```python
from build123d import *

# Parameters (mm, degrees)
SKETCH_W              = 115
SKETCH_H              = 25
PAD_DEPTH             = 3
PAD001_DEPTH          = 3
SKETCH002_W           = 115
SKETCH002_H           = 25
SKETCH002_W_2         = 96
SKETCH002_H_2         = 3
PAD002_DEPTH          = 3
SKETCH003_R           = 0.825
POCKET_DEPTH          = 245.060315
POLARPATTERN_COUNT    = 2
POLARPATTERN001_COUNT = 2
POLARPATTERN002_COUNT = 2
FILLET_R              = 2
SKETCH004_R           = 12.75
POCKET001_DEPTH       = 3
POCKET002_DEPTH       = 3


with BuildPart() as part:
    # Sketch → Pad (new body)
    with BuildSketch(Plane.XY):
        Rectangle(SKETCH_W, SKETCH_H)
    extrude(amount=PAD_DEPTH)

    # Sketch001 (on Face6 of Pad) → Pad001 (join)
    with BuildSketch(Plane.XY.offset(3)):
        Polygon((-57.5, 12.5), (57.5, 12.5), (57.5, 4), (50, 4), (50, 5), (-50, 5), (-50, 4), (-57.5, 4), align=None)
        Polygon((-57.5, -12.5), (57.5, -12.5), (57.5, -4), (50, -4), (50, -5), (-50, -5), (-50, -4), (-57.5, -4), align=None)
    extrude(amount=PAD001_DEPTH)

    # Sketch002 (on Face12 of Pad001) → Pad002 (join)
    with BuildSketch(Plane.XY.offset(6)):
        Rectangle(SKETCH002_W, SKETCH002_H)
        Rectangle(SKETCH002_W_2, SKETCH002_H_2, mode=Mode.SUBTRACT)
    extrude(amount=PAD002_DEPTH)

    # Sketch003 (on Face26 of Pad002) → Pocket (cut, through all)
    with BuildSketch(Plane.XY.offset(9)):
        with Locations((-52.5, 7.5)):
            Circle(SKETCH003_R)
    pocket = extrude(amount=-POCKET_DEPTH, mode=Mode.SUBTRACT)

    # PolarPattern: Pocket ×2 about axis
    polarpattern_axis = Axis((0, 0, 0), (0, 1, 0))
    for i in range(1, POLARPATTERN_COUNT):
        add(pocket.rotate(polarpattern_axis, i * 360 / POLARPATTERN_COUNT), mode=Mode.SUBTRACT)

    # PolarPattern001: Pocket ×2 about axis
    polarpattern001_axis = Axis((0, 0, 0), (1, 0, 0))
    for i in range(1, POLARPATTERN001_COUNT):
        add(pocket.rotate(polarpattern001_axis, i * 360 / POLARPATTERN001_COUNT), mode=Mode.SUBTRACT)

    # PolarPattern002: Pocket ×2 about axis
    polarpattern002_axis = Axis((0, 0, 9), (0, 0, 1))
    for i in range(1, POLARPATTERN002_COUNT):
        add(pocket.rotate(polarpattern002_axis, i * 360 / POLARPATTERN002_COUNT), mode=Mode.SUBTRACT)

    # Fillet
    fillet_edges = [part.edges().sort_by_distance(p)[0] for p in [
        (57.5, 12.5, 7.5),
        (57.5, 12.5, 4.5),
        (57.5, 12.5, 1.5),
        (57.5, -12.5, 7.5),
        (-57.5, 12.5, 7.5),
        (-57.5, -12.5, 7.5),
    ]]
    fillet(fillet_edges, radius=FILLET_R)

    # Sketch004 (on Face2 of Fillet) → Pocket001 (cut)
    with BuildSketch(Plane(origin=(0, 0, 0), x_dir=(1, 0, 0), z_dir=(0, 0, -1))):
        with Locations((0, -4.31247)):
            Circle(SKETCH004_R)
    extrude(amount=-POCKET001_DEPTH, mode=Mode.SUBTRACT)

    # Sketch005 (on Face2 of Pocket001) → Pocket002 (cut)
    with BuildSketch(Plane(origin=(0, 0, 0), x_dir=(1, 0, 0), z_dir=(0, 0, -1))):
        Polygon((0.086598, 10.584693), (-49.736099, 10.584693), (-49.736099, 6.30074), (-54.94091, 3.161258), (-54.94091, -2.621142), (-51.300568, -2.835279), (-51.086433, 1.161956), (-44.025761, 5.729707), (0.086598, 5.729707), align=None)
    extrude(amount=-POCKET002_DEPTH, mode=Mode.SUBTRACT)


solid = part.part
```
The model under review builds one solid part; all positions refer to its coordinate system, in mm. A direction names the side the tool comes from. Coordinates: 2 decimals unless noted, no trailing zeros. Write each loop counter-clockwise with the first axis right and the second up, starting at its lowest first coordinate (ties: lowest second). Pieces come first, ordered by that corner, then holes. Notation, with made-up numbers: (-13.5, 77) - (-5.5, 77) arc R25 cw to (-5.5, 111) - close; hole circle Ø4 at (84.5, 31.25). An arc over 180 degrees is marked (long way). Answer in a Markdown table with one row per item. Add a question column.
Q1. Consider section C-C on z = 1.25. Give the boundary of the cut face in (x, y) (3 decimals).
Q2. Clearance check with a flat-ended pin moving along its axis: pin 1 (6 mm diameter, centred on x = 5.5, y = 7.5, fed in from -Z). State where the tip first meets the part, or that it passes through.
Q3. Draft analysis for pull direction X (two halves, no side actions). For faces 6 (the face through (0, 9, 3)), 7 (the face through (-56.93, 11.9, 4.44)), 8 (the face through (-1, -12.5, 4)), state which applies: +X half, -X half, draft (parallel to the pull), parting line (faces both ways), or undercut.
Q4. Consider section A-A on z = 8. Give the boundary of the cut face in (x, y) (3 decimals), then the cut area to 3 significant figures.
Q5. Consider section B-B on x = -23. Give the boundary of the cut face in (y, z).
Q6. To check wall thickness, follow line 1 along Y through (x, z) = (-52.5, 3.5) (3 decimals); line 2 along Y through (x, z) = (-52.5, 6.5) (3 decimals); line 3 along Z through (x, y) = (-39, 3.5). State the ranges of each line that lie inside material, in increasing order. Write a range as from..to.
Q7. For faces 1 (the face through (-52.302, -4.753, 1.479)), 2 (the face through (-33, 0, 3)), 3 (the face through (-57.5, -0.1, 6.4)), 4 (the face through (-54, -4, 4)), 5 (the face through (-1, -1.5, 7)), list the 3-axis set-ups (+Z, -Z, +X, -X, +Y, -Y) from which the entire face can be reached by the end or side of a thin tool; tool diameter is ignored.
Answers below:
| question | item | result |
|---|---|---|
| 1 | outline | (-57.5, -10.5) arc R2 ccw to (-55.5, -12.5) - (55.5, -12.5) arc R2 ccw to (57.5, -10.5) - (57.5, 10.5) arc R2 ccw to (55.5, 12.5) - (9.774, 12.5) arc R12.75 cw to (0.087, -8.437) - (0.087, -10.585) - (-49.736, -10.585) - (-49.736, -6.301) - (-54.941, -3.161) - (-54.941, 2.621) - (-51.301, 2.835) - (-51.086, -1.162) - (-44.026, -5.73) - (-7.856, -5.73) arc R12.75 cw to (-9.774, 12.5) - (-55.5, 12.5) arc R2 ccw to (-57.5, 10.5) - close; hole circle Ø1.65 at (-52.5, -7.5); hole circle Ø1.65 at (-52.5, 7.5); hole circle Ø1.65 at (52.5, -7.5); hole circle Ø1.65 at (52.5, 7.5) |
| 2 | pin 1 | z = 3 |
| 3 | face 6 | undercut |
| 3 | face 7 | -X half |
| 3 | face 8 | draft |
| 4 | outline | (-57.5, -10.5) arc R2 ccw to (-55.5, -12.5) - (55.5, -12.5) arc R2 ccw to (57.5, -10.5) - (57.5, 10.5) arc R2 ccw to (55.5, 12.5) - (-55.5, 12.5) arc R2 ccw to (-57.5, 10.5) - close; hole circle Ø1.65 at (-52.5, -7.5); hole circle Ø1.65 at (-52.5, 7.5); hole (-48, -1.5) - (48, -1.5) - (48, 1.5) - (-48, 1.5) - close; hole circle Ø1.65 at (52.5, -7.5); hole circle Ø1.65 at (52.5, 7.5) |
| 4 | area | 2,580 mm² |
| 5 | outline | (-12.5, 0) - (-10.58, 0) - (-10.58, 3) - (-5.73, 3) - (-5.73, 0) - (12.5, 0) - (12.5, 9) - (1.5, 9) - (1.5, 6) - (5, 6) - (5, 3) - (-5, 3) - (-5, 6) - (-1.5, 6) - (-1.5, 9) - (-12.5, 9) - close |
| 6 | line 1 | -12.5..-8.325, -6.675..-4, 4..6.675, 8.325..12.5 |
| 6 | line 2 | -12.5..-8.325, -6.675..6.675, 8.325..12.5 |
| 6 | line 3 | 0..3, 6..9 |
| 7 | face 1 | -Z |
| 7 | face 2 | none |
| 7 | face 3 | +Z, -Z, -X, +Y, -Y |
| 7 | face 4 | +X, -X |
| 7 | face 5 | +Z |
